Input: part model. Units: mm. Frame: model coordinates. A direction names the side the tool comes from. Coordinates: 2 decimals unless noted, no trailing zeros. Loops run counter-clockwise (first coordinate to the right, second up) from the corner with the lowest first, then second, coordinate; pieces in that order, holes last. Notation, with made-up numbers: (17, 0.5) - (24, 0.5) arc R15 cw to (24, 8.5) - close; hole circle Ø3 at (44.5, -24.75). An arc over 180 degrees is marked (long way). Use a Markdown table: item, result. Add a question column.
1. Contact query for flat-ended pins moving along their axis: P1, Ø2.5, axis at x = 7.5, z = 1, coming from the -Y side; P2, Ø3, axis at x = 5.5, z = 1, coming from the +Y side; P3, Ø5, axis at y = 2.5, z = -2.5, coming from the +X side; P4, Ø6, axis at y = 2, z = -1.5, coming from the -X side. Output: stop coordinate, or through.
2. Section query C-C on z = 5. Return the cut outline in (x, y), then the cut area to 3 significant figures.
3. Section query B-B on y = 2. Return the cut outline in (x, z).
4. Draft query along Z for faces 1 (the face through (5, 0, -4.25)), 2 (the face through (12.197, -7.49, 5.264)), 3 (the face through (5, 0, -6.25)), 4 (the face through (15, 0, 4.25)). Return one class per face: released by +Z, released by -Z, zero draft, split by the parting line, or undercut.
5. Section query D-D on x = 17.5. Return the cut outline in (y, z), then the cut area to 3 significant figures.
6. Access query for faces 5 (the face through (10, -0.1, -4.4)), 6 (the face through (5, -3.05, 0)), 7 (the face through (0, -3.4, 0.1)). Directions: +Z, -Z, +X, -X, +Y, -Y. A direction counts if a zero-diameter tool reaches every point of the face in a straight line with its end or side. Return the directions, or none.
7. Ray query, L1, parallel to Z at x = 8, y = 2.5; L2, parallel to Y at x = 4.75, z = 3.5; L3, parallel to Z at x = 20.5, y = 8.5. Return the intervals inside material, ascending. Write a range as [from, to].
8. Section query A-A on z = 1.25. Return the cut outline in (x, y), then the cut area to 3 significant figures.
```python
from build123d import *

# Parameters (mm, degrees)
F0_W        = 10.1
F0_H        = 12.5
F0_W_2      = 6.1
F0_H_2      = 8.5
F1_DEPTH    = 10
F2_W        = 15
F2_H        = 2
F3_DEPTH    = 10
F4_T4_DEPTH = 27.7168298797
F4_T9_DEPTH = 27.7168298797


# Not quite as in the source:
# - a fillet or chamfer that OpenCascade refuses, or shapes differently, is made with other operations: its cross-section is extruded or revolved along the edge and cut away or added


with BuildPart() as f1:
    # F0 (on Right) → F1 (new body)
    with BuildSketch(Plane.YZ):
        Rectangle(F0_W, F0_H)
        Rectangle(F0_W_2, F0_H_2, mode=Mode.SUBTRACT)
    extrude(amount=F1_DEPTH)

    # F2 (on Front) → F3 (join, symmetric)
    with BuildSketch(Plane.XZ):
        with Locations((17.2066340968, 5.25)):
            Rectangle(F2_W, F2_H)
    extrude(amount=F3_DEPTH, both=True)

    # F4: chamfer of 5 on 2 edges, made by hand


with BuildPart() as f4_tool2:
    # F4_s3 → F4_t4 (new body)
    with BuildSketch(Plane.XY.offset(19.1084149398)):
        Polygon((14.7066340968, 10), (9.7066340968, 5), (9.7066340968, 10), align=None)
    extrude(amount=-F4_T4_DEPTH)

    split(bisect_by=Plane.XZ.offset(-5.05), keep=Keep.BOTTOM)


with BuildPart() as f1_1:
    add(f1.part)

    # F4_t1: cut F4_tool2
    add(f4_tool2.part, mode=Mode.SUBTRACT)


with BuildPart() as f4_tool7:
    # F4_s8 → F4_t9 (new body)
    with BuildSketch(Plane.XY.offset(19.1084149398)):
        Polygon((9.7066340968, -5), (14.7066340968, -10), (9.7066340968, -10), align=None)
    extrude(amount=-F4_T9_DEPTH)

    split(bisect_by=Plane.XZ.offset(5.05), keep=Keep.TOP)


with BuildPart() as f1_2:
    add(f1_1.part)

    # F4_t6: cut F4_tool7
    add(f4_tool7.part, mode=Mode.SUBTRACT)


solid = f1_2.part
```
Resolved:
| question | item | result |
|---|---|---|
| 1 | P1 | y = -5.05 |
| 1 | P2 | y = 5.05 |
| 1 | P3 | x = 10 |
| 1 | P4 | x = 0 |
| 2 | outline | (0, -5.05) - (9.76, -5.05) - (14.71, -10) - (24.71, -10) - (24.71, 10) - (14.71, 10) - (9.76, 5.05) - (0, 5.05) - close |
| 2 | area | 373 mm² |
| 3 | outline | (0, -6.25) - (10, -6.25) - (10, -4.25) - (0, -4.25) - close; (0, 4.25) - (24.71, 4.25) - (24.71, 6.25) - (0, 6.25) - close |
| 4 | face 1 | undercut |
| 4 | face 2 | zero draft |
| 4 | face 3 | released by -Z |
| 4 | face 4 | undercut |
| 5 | outline | (-10, 4.25) - (10, 4.25) - (10, 6.25) - (-10, 6.25) - close |
| 5 | area | 40.0 mm² |
| 6 | face 5 | -Z, +X, +Y, -Y |
| 6 | face 6 | +X, -X |
| 6 | face 7 | +Z, -Z, -X, +Y, -Y |
| 7 | L1 | [-6.25, -4.25], [4.25, 6.25] |
| 7 | L2 | [-5.05, -3.05], [3.05, 5.05] |
| 7 | L3 | [4.25, 6.25] |
| 8 | outline | (0, -5.05) - (10, -5.05) - (10, -3.05) - (0, -3.05) - close; (0, 3.05) - (10, 3.05) - (10, 5.05) - (0, 5.05) - close |
| 8 | area | 40.0 mm² |
